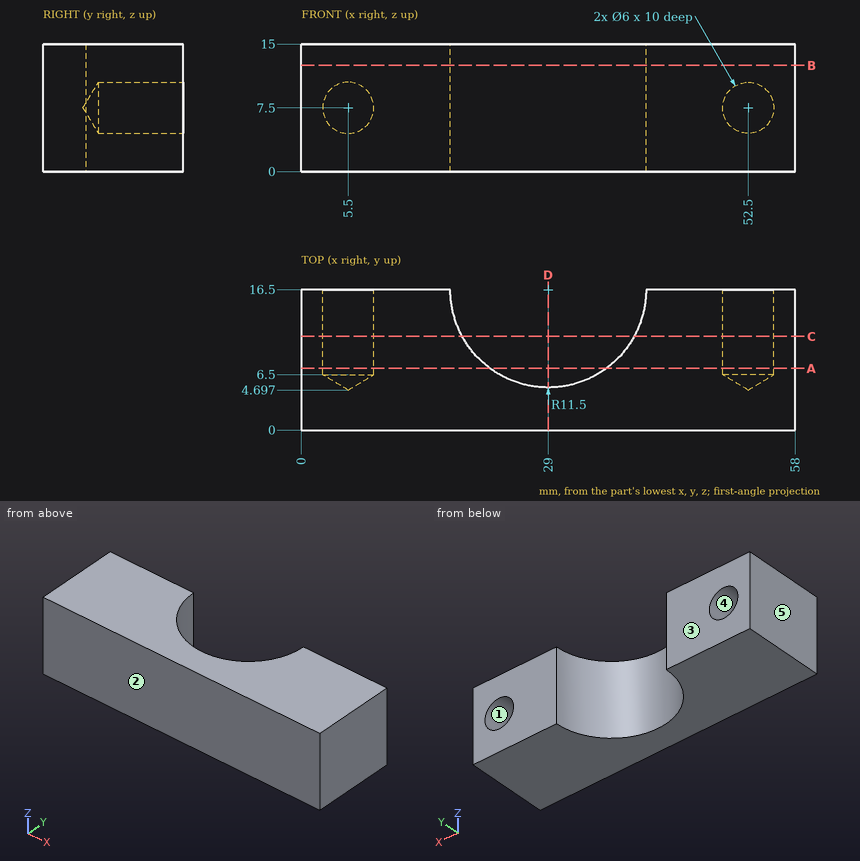
Design review of the part shown in the three views and the two pictorial views. Dimensions are in mm from the part's minimum x, y and z. A direction names the side the tool comes from. Round coordinates to 2 decimals unless told otherwise and drop trailing zeros. Loops run counter-clockwise (first coordinate to the right, second up) from the corner with the lowest first, then second, coordinate; pieces in that order, holes last. Notation, with made-up numbers: (62, 73) - (110, 73) arc R31 ccw to (110, 102) - close; hole circle Ø6 at (89, -21). An arc over 180 degrees is marked (long way). One line per item, written item: value. Start each with the question number.
Item 1: The part is to be moulded in two halves that separate along X. For the marked faces 3, 4 and 5, say which applies: +X half, -X half, draft (parallel to the pull), parting line (faces both ways), or undercut.
Item 2: Take a section at D-D (x = 29). Give the boundary of the cut face in (y, z).
Item 3: Take a section at B-B (z = 12.5). Give the boundary of the cut face in (x, y).
Item 4: Take a section at C-C (y = 11). Give the boundary of the cut face in (x, z).
Item 5: For L1, parallel to Z at x = 5.5, y = 14.25; L2, parallel to X at y = 9.5, z = 7.5 (1 decimal); L3, parallel to X at y = 11.75, z = 5.5 (1 decimal), list the stretches that pass through material, from the lowest coordinate up.
Item 6: Take a section at A-A (y = 7.25). Give the boundary of the cut face in (x, z).
Item 7: For the marked faces 1 and 2, list the 3-axis set-ups (+Z, -Z, +X, -X, +Y, -Y) from which the entire face can be reached by the end or side of a thin tool; tool diameter is ignored.
Answer below:
1. face 3: draft
1. face 4: undercut
1. face 5: -X half
2. outline: (0, 0) - (5, 0) - (5, 15) - (0, 15) - close
3. outline: (0, 0) - (58, 0) - (58, 16.5) - (40.5, 16.5) arc R11.5 cw to (17.5, 16.5) - (0, 16.5) - close
4. outline: (0, 0) - (18.9, 0) - (18.9, 15) - (0, 15) - close; (39.1, 0) - (58, 0) - (58, 15) - (39.1, 15) - close; hole circle Ø6 at (5.5, 7.5); hole circle Ø6 at (52.5, 7.5)
5. L1: z = 0 to 4.5, 10.5 to 15
5. L2: x = 0 to 2.5, 8.5 to 19.9, 38.1 to 49.5, 55.5 to 58
5. L3: x = 0 to 3.3, 7.7 to 18.5, 39.5 to 50.3, 54.7 to 58
6. outline: (0, 0) - (22.17, 0) - (22.17, 15) - (0, 15) - close; (35.83, 0) - (58, 0) - (58, 15) - (35.83, 15) - close; hole circle Ø6 at (5.5, 7.5); hole circle Ø6 at (52.5, 7.5)
7. face 1: +Y
7. face 2: +Z, -Z, +X, -X, -Y
